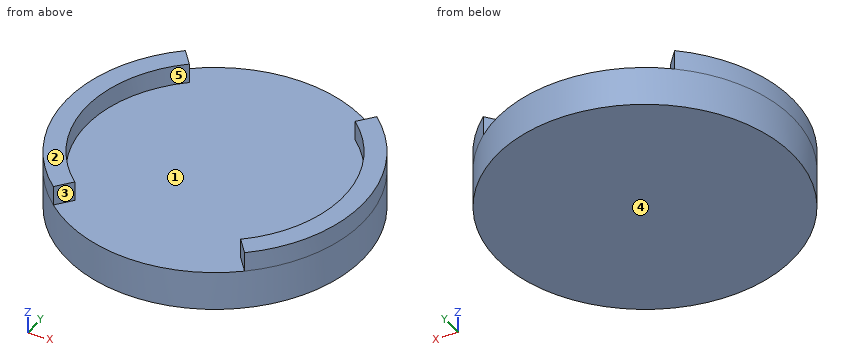
from build123d import *

# Parameters (mm, degrees)
F0_R     = 19.05
F1_DEPTH = 5.08
F3_DEPTH = 2.54


# Not quite as in the source:
# - a pattern or mirror of a feature is missing from the dataset's text; its kind, count and spacing are read off the source's solid


with BuildPart() as f1:
    # F0 (on Top) → F1 (new body)
    with BuildSketch(Plane.XY):
        Circle(F0_R)
    extrude(amount=F1_DEPTH)

    # F2 (on face) → F3 (join)
    with BuildSketch(Plane.XY.offset(5.08)):
        with BuildLine():
            ThreePointArc((-10.6124234359, -12.6473937559), (-16.51, 0), (-10.6124234359, 12.6473937559))
            Line((-10.6124234359, 12.6473937559), (-12.2451039645, 14.5931466414))
            ThreePointArc((-12.2451039645, 14.5931466414), (-19.05, 0), (-12.2451039645, -14.5931466414))
            Line((-12.2451039645, -14.5931466414), (-10.6124234359, -12.6473937559))
        make_face()
    f3 = extrude(amount=F3_DEPTH)

    # F3_copies: F3 across plane
    add(f3.mirror(Plane(origin=(0, 0, 0), x_dir=(0, 0, 1), z_dir=(1, 0, 0))))


solid = f1.part
Source: CAD feature listing. Evaluate the final solid. Frame: model axes, mm. Face numbers are marked on the shaded views. A direction names the side the tool comes from. Round coordinates to 2 decimals unless told otherwise and drop trailing zeros. Loops run counter-clockwise (first coordinate to the right, second up) from the corner with the lowest first, then second, coordinate; pieces in that order, holes last. Notation, with made-up numbers: M 39,10.25 L 53,10.25 A25 cw 53,49.25 Z; hole C 77.5,-28.75 d9. An arc over 180 degrees is marked long. Return JSON: item names as keys, results as strings. Group by question number.
1. Material intervals for line 1 along X through (y, z) = (-14, 6); line 2 along Z through (x, y) = (3, -9); line 3 along X through (y, z) = (3, 7), sorted ascending. Write a range as from..to.
2. Section query D-D on z = 4. Output: boundary loops of the cut face in (x, y), and give its area (3 significant figures).
3. Mould query, pull axis Y, two halves, no side actions, for the marked faces 3, 4 and 5. Classes: released by +Y, released by -Y, zero draft, split by the parting line, or undercut.
4. Section query C-C on x = -13. Output: boundary loops of the cut face in (y, z), and give its area (3 significant figures).
5. Reachability of the marked faces 1 and 2 from +Z, -Z, +X, -X, +Y, -Y: full face, straight path, thin tool, end or side. Return the list, or none.
6. Pin query (flat end, axial travel): pin 1 (3 mm diameter, centred on x = -5.5, z = 1.5, fed in from -Y); pin 2 (2 mm diameter, centred on y = -5, z = 1, fed in from -X); pin 3 (2 mm diameter, centred on y = -6.5, z = 1, fed in from -X). Return the tip coordinate at first contact, or that it passes through.
7. Section query B-B on y = 0. Output: boundary loops of the cut face in (x, z), and give its area (3 significant figures).
8. Section query A-A on z = 6.25. Output: boundary loops of the cut face in (x, y), and give its area (3 significant figures).
Checks:
{
 "1": {"line 1": "x = -12.92..-11.75, 11.75..12.92", "line 2": "z = 0..5.08", "line 3": "x = -18.81..-16.24, 16.24..18.81"},
 "2": {"outline": "C 0,0 d38.1", "area": "1,140 mm²"},
 "3": {"face 3": "released by -Y", "face 4": "zero draft", "face 5": "undercut"},
 "4": {"outline": "M -13.92,0 L 13.92,0 L 13.92,7.62 L 10.18,7.62 L 10.18,5.08 L -10.18,5.08 L -10.18,7.62 L -13.92,7.62 Z", "area": "161 mm²"},
 "5": {"face 1": "+Z", "face 2": "+Z, +X, -X, +Y, -Y"},
 "6": {"pin 1": "stops at y = -18.63", "pin 2": "stops at x = -18.63", "pin 3": "stops at x = -18.24"},
 "7": {"outline": "M -19.05,0 L 19.05,0 L 19.05,7.62 L 16.51,7.62 L 16.51,5.08 L -16.51,5.08 L -16.51,7.62 L -19.05,7.62 Z", "area": "206 mm²"},
 "8": {"outline": "M -12.25,-14.59 L -10.61,-12.65 A16.51 cw -10.61,12.65 L -12.25,14.59 A19.05 ccw Z; M 10.61,-12.65 L 12.25,-14.59 A19.05 ccw 12.25,14.59 L 10.61,12.65 A16.51 cw Z", "area": "158 mm²"}
}
